Model file for the job. Use its own axes, mm. A direction names the side the tool comes from. Give positions to 0.01 mm unless a question says otherwise; leave off trailing zeros. Write each loop counter-clockwise with the first axis right and the second up, starting at its lowest first coordinate (ties: lowest second). Pieces come first, ordered by that corner, then holes.
```python
from build123d import *

# Parameters (mm, degrees)
F0_W     = 900
F0_H     = 1200
F1_DEPTH = 50
F3_DEPTH = 100


# Not quite as in the source:
# - the program builds the solid bodies; features that only make, move or delete a surface that nothing else refers to are left out


with BuildPart() as f1:
    # F0 (on Top) → F1 (new body)
    with BuildSketch(Plane.XY):
        Rectangle(F0_W, F0_H)
    extrude(amount=-F1_DEPTH)

    # F2 (on face) → F3 (join)
    with BuildSketch(Plane.XY):
        with BuildLine():
            Line((-400.0000059605, -525), (-400.0000059605, -550))
            Line((-400.0000059605, -550), (-375.0000059605, -550))
            ThreePointArc((-375.0000059605, -550), (-382.3223364308, -532.3223304703), (-400.0000059605, -525))
        make_face()
        with BuildLine():
            ThreePointArc((-400.0000059605, -525), (-382.3223364308, -532.3223304703), (-375.0000059605, -550))
            Line((-375.0000059605, -550), (375, -550))
            ThreePointArc((375, -550), (382.3223304703, -532.3223304703), (400, -525))
            Line((400, -525), (400, 550))
            Line((400, 550), (-400.0000059605, 550))
            Line((-400.0000059605, 550), (-400.0000059605, -525))
        make_face()
        with BuildLine():
            ThreePointArc((400, -525), (382.3223304703, -532.3223304703), (375, -550))
            Line((375, -550), (400, -550))
            Line((400, -550), (400, -525))
        make_face()
    extrude(amount=F3_DEPTH)


solid = f1.part
```
1. Pin check, flat tips, straight feed: P1, Ø2, axis at y = -232, z = 49, coming from the -X side; P2, Ø6, axis at x = 71, z = 5, coming from the +Y side; P3, Ø3, axis at x = 45.5, z = 81, coming from the -Y side. Stop position of each tip, or through.
Calculated:
P1: stops at x = -400
P2: stops at y = 550
P3: stops at y = -550
2. Slice it at C-C, the plane z = 13.5. Write the cut outline in (x, y), and give its area (3 significant figures).
Calculated:
outline: (-400, -550) - (400, -550) - (400, 550) - (-400, 550) - close
area: 880,000 mm2
3. Which spindle directions (+Z, -Z, +X, -X, +Y, -Y) get a long thin tool onto all of the face, cutting with end or side? Do faces 1 (the flat face through (-6, -550, 49)), 2 (the flat face through (-400, 8, 49)), 3 (the flat face through (6, 550, 49)), 4 (the flat face through (-6, 8, 100)), 5 (the flat face through (400, -8, 49)). Say none if no direction does.
Calculated:
face 1: +Z, +X, -X, -Y
face 2: +Z, -X, +Y, -Y
face 3: +Z, +X, -X, +Y
face 4: +Z, +X, -X, +Y, -Y
face 5: +Z, +X, +Y, -Y
4. Slice it at B-B, the plane y = 425. Write the cut outline in (x, z).
Calculated:
outline: (-450, -50) - (450, -50) - (450, 0) - (400, 0) - (400, 100) - (-400, 100) - (-400, 0) - (-450, 0) - close
5. Slice it at A-A, the plane x = -82. Write the cut outline in (y, z), and give its area (3 significant figures).
Calculated:
outline: (-600, -50) - (600, -50) - (600, 0) - (550, 0) - (550, 100) - (-550, 100) - (-550, 0) - (-600, 0) - close
area: 170,000 mm2
6. Probe probe 1 along X at (y, z) = (-299, 10); probe 2 along Y at (x, z) = (-13.5, 55); probe 3 along Z at (x, y) = (-401.5, -195). List the from-to ranges inside material, lowest first.
Calculated:
probe 1: x = -400 to 400
probe 2: y = -550 to 550
probe 3: z = -50 to 0
